Verification items for the finished model (mm, model axes). A direction names the side the tool comes from. Give positions to 0.01 mm unless a question says otherwise; leave off trailing zeros. Write each loop counter-clockwise with the first axis right and the second up, starting at its lowest first coordinate (ties: lowest second). Pieces come first, ordered by that corner, then holes. Notation, with made-up numbers: M 34.25,72 L 76.25,72 A33 cw 76.25,101 Z; hole C 39,-30.5 d9. An arc over 180 degrees is marked long. Answer as a JSON object with one key per item and string values.
```python
from build123d import *

# Parameters (mm, degrees)
F0_R     = 20.32
F1_DEPTH = 2.54
F2_R     = 3.4925
F3_DEPTH = 25.4
F5_DEPTH = 1.524


with BuildPart() as f1:
    # F0 (on Front) → F1 (new body)
    with BuildSketch(Plane.XZ):
        Circle(F0_R)
    extrude(amount=F1_DEPTH)

    # F2 (on face) → F3 (cut)
    with BuildSketch(Plane.XZ.offset(2.54)):
        Circle(F2_R)
    extrude(amount=-F3_DEPTH, mode=Mode.SUBTRACT)

    # F4 (on face) → F5 (cut)
    with BuildSketch(Plane.XZ.offset(2.54)):
        Polygon((14.7066, 1.9939), (2.224531, 2.6924), (2.224531, -2.6924), (14.7066, -1.9939), (16.256, -0.993628), (16.256, 1.051273), align=None)
    extrude(amount=-F5_DEPTH, mode=Mode.SUBTRACT)


solid = f1.part
```
1) Section check A-A on x = 0. Record the boundary of the cut face in (y, z), and give its area (3 significant figures).
Completed:
{"outline": "M -2.54,-20.32 L 0,-20.32 L 0,-3.49 L -2.54,-3.49 Z; M -2.54,3.49 L 0,3.49 L 0,20.32 L -2.54,20.32 Z", "area": "85.5 mm2"}
2) Section check D-D on x = 8. Record the boundary of the cut face in (y, z), and give its area (3 significant figures).
Completed:
{"outline": "M -2.54,-18.68 L 0,-18.68 L 0,18.68 L -2.54,18.68 L -2.54,2.37 L -1.02,2.37 L -1.02,-2.37 L -2.54,-2.37 Z", "area": "87.7 mm2"}
3) Thickness scan on L1, parallel to Z at x = 0, y = -1.1; L2, parallel to Z at x = -3, y = -0.7; L3, parallel to X at y = -1.3, z = -1.5. Record the ranges inside material, lowest first.
Completed:
{"L1": "z = -20.32 to -3.49, 3.49 to 20.32", "L2": "z = -20.1 to -1.79, 1.79 to 20.1", "L3": "x = -20.26 to -3.15, 15.47 to 20.26"}
4) Section check C-C on z = 0. Record the boundary of the cut face in (x, y).
Completed:
{"outline": "M -20.32,-2.54 L -3.49,-2.54 L -3.49,0 L -20.32,0 Z; M 3.49,-1.02 L 16.26,-1.02 L 16.26,-2.54 L 20.32,-2.54 L 20.32,0 L 3.49,0 Z"}
5) Release check for a two-part mould opening along Z. For faces 1 (the face through (-2.645, -1.252, 20.147)), 2 (the face through (0, -2.54, -4)), 3 (the face through (-3.49, -1.29, 0.15)) record: pulls with the +Z half, pulls with the -Z half, needs draft (parallel to the pull), parting line crosses it, or undercut.
Completed:
{"face 1": "parting line crosses it", "face 2": "needs draft", "face 3": "undercut"}
6) Access from +Z, -Z, +X, -X, +Y, -Y to the whole of each face (thin tool, end or side, straight path). Record for faces 4 (the face through (4, 0, 0)), 5 (the face through (15.47, -1.79, -1.5)).
Completed:
{"face 4": "+Z, -Z, +X, -X, +Y", "face 5": "-Y"}
7) Section check B-B on y = -2.15. Record the boundary of the cut face in (x, z) (1 decimal), and give its area (3 significant figures).
Completed:
{"outline": "C 0,0 d40.6; hole M 2.2,-2.7 L 14.7,-2 L 16.3,-1 L 16.3,1.1 L 14.7,2 L 2.2,2.7 A3.5 ccw long Z", "area": "1,200 mm2"}
